The listing builds one solid part. Answer for the finished solid, in the listing's coordinates (mm). Face numbers are marked on the shaded views. A direction names the side the tool comes from. Coordinates: 2 decimals unless noted, no trailing zeros. Loops run counter-clockwise (first coordinate to the right, second up) from the corner with the lowest first, then second, coordinate; pieces in that order, holes last. Notation, with made-up numbers: (86, 74.5) - (136, 74.5) arc R18 cw to (136, 88.5) - close; hole circle Ø4 at (63.5, -26). An arc over 180 degrees is marked (long way). Write each question's results on one line, items separated by ' | '. Start each with the question number.
(1) Find section C-C on x = 7. Determine the outline of the cut face in (y, z), then the cut area to 3 significant figures.
(2) Find section A-A on y = 0. Determine the outline of the cut face in (x, z), then the cut area to 3 significant figures.
(3) Given pin 1 Ø12 at (x, y) = (-7, 30) entering from -Z; pin 2 Ø6 at (x, y) = (0, 35.5) entering from +Z; pin 3 Ø7 at (x, y) = (-17, 27.5) entering from +Z; pin 4 Ø3.5 at (x, y) = (-17, -27.5) entering from +Z, each flat-ended and moving along its own axis, determine where each tip first touches the part or whether it passes through.
(4) Consider line 1 (X direction, y = -27.5, z = 1.45); line 2 (Y direction, x = -27, z = -3.5); line 3 (Z direction, x = -29, y = -26.5). Determine where each line is inside the solid, lowest interval first. Write a range as from..to.
(5) Find section D-D on y = -17.75. Determine the outline of the cut face in (x, z), then the cut area to 3 significant figures.
(6) For the marked faces 1, 2 and 3, determine the directions among +Z, -Z, +X, -X, +Y, -Y from which every point of the face is accessible in a straight line to the end or side of a thin tool.
(7) Find section B-B on x = -17. Determine the outline of the cut face in (y, z).
(8) Determine the mould class of the marked faces 4, 5 and 6 for opening direction Y: released by +Y, released by -Y, zero draft, split by the parting line, or undercut.
from build123d import *

# Parameters (mm, degrees)
SKETCH_1_W                     = 80
SKETCH_1_H                     = 80
SKETCH_1_R                     = 25
EXTRUDE_1_DEPTH                = 6
SKETCH_11_W                    = 10
SKETCH_11_H                    = 10
EXTRUDE_3_DEPTH                = 10
HOLE_WIZARD_M4_1_D             = 4.5
HOLE_WIZARD_M4_1_CSINK_D       = 8.96
HOLE_WIZARD_M4_1_CSINK_ANGLE   = 90
HOLE_WIZARD_M4_2_D             = 3.3
HOLE_WIZARD_M4_2_DEPTH         = 68
MIRROR_2_COPY_1_SKETCH_W       = 10
MIRROR_2_COPY_1_SKETCH_H       = 10
MIRROR_2_COPY_1_DEPTH          = 10
MIRROR_2_COPY_2_D              = 3.3
MIRROR_2_COPY_2_DEPTH          = 68
HOLE_WIZARD_M4_1_2_D           = 4.5
HOLE_WIZARD_M4_1_2_CSINK_D     = 9.4
HOLE_WIZARD_M4_1_2_CSINK_ANGLE = 90
CHAMFER_1_SIZE                 = 1


with BuildPart() as part:
    # 스케치1 → 보스-돌출1 (new body)
    with BuildSketch(Plane.XY):
        Rectangle(SKETCH_1_W, SKETCH_1_H)
        Circle(SKETCH_1_R, mode=Mode.SUBTRACT)
    extrude(amount=EXTRUDE_1_DEPTH)

    # 스케치11 → 보스-돌출3 (add)
    with BuildSketch(Plane(origin=(0, 0, 0), x_dir=(-1, 0, 0), z_dir=(0, 0, -1))):
        with Locations((29, 29)):
            Rectangle(SKETCH_11_W, SKETCH_11_H)
    extrude_3 = extrude(amount=EXTRUDE_3_DEPTH)

    # Hole Wizard M4 _ _ _ _ _ _ _1 (through all)
    with Locations(Plane(origin=(0, 0, 0), x_dir=(-1, 0, 0), z_dir=(0, 0, -1))):
        with Locations((0, -35.5), (30.743901834, -17.75), (30.743901834, 17.75), (0, 35.5), (-30.743901834, 17.75), (-30.743901834, -17.75)):
            CounterSinkHole(HOLE_WIZARD_M4_1_D / 2, HOLE_WIZARD_M4_1_CSINK_D / 2, counter_sink_angle=HOLE_WIZARD_M4_1_CSINK_ANGLE)

    # M4 나사 구멍2
    with Locations(Plane(origin=(0, 34, 0), x_dir=(1, 0, 0), z_dir=(0, 1, 0))):
        with Locations((-29, 5)):
            hole_wizard_m4_2 = Hole(HOLE_WIZARD_M4_2_D / 2, depth=HOLE_WIZARD_M4_2_DEPTH)

    # 대칭 복사1: 보스-돌출3, M4 나사 구멍2 across plane
    add(extrude_3.mirror(Plane(origin=(0, 0, 0), x_dir=(0, 0, 1), z_dir=(1, 0, 0))))
    add(hole_wizard_m4_2.mirror(Plane(origin=(0, 0, 0), x_dir=(0, 0, 1), z_dir=(1, 0, 0))), mode=Mode.SUBTRACT)

    # 대칭 복사2: 보스-돌출3, M4 나사 구멍2 across plane
    add(extrude_3.mirror(Plane.ZX))
    add(hole_wizard_m4_2.mirror(Plane.ZX), mode=Mode.SUBTRACT)

    # 대칭 복사2 copy 1 sketch → 대칭 복사2 copy 1 (add)
    with BuildSketch(Plane(origin=(0, 0, 0), x_dir=(1, 0, 0), z_dir=(0, 0, -1))):
        with Locations((29, 29)):
            Rectangle(MIRROR_2_COPY_1_SKETCH_W, MIRROR_2_COPY_1_SKETCH_H)
    extrude(amount=MIRROR_2_COPY_1_DEPTH)

    # 대칭 복사2 copy 2
    with Locations(Plane(origin=(0, -34, 0), x_dir=(-1, 0, 0), z_dir=(0, -1, 0))):
        with Locations((-29, 5)):
            Hole(MIRROR_2_COPY_2_D / 2, depth=MIRROR_2_COPY_2_DEPTH)

    # Hole Wizard M4 _ _ _ _1 2 (through all)
    with Locations(Plane.XY.offset(6)):
        with Locations((17, 27.5), (17, -27.5), (-17, 27.5), (-17, -27.5)):
            CounterSinkHole(HOLE_WIZARD_M4_1_2_D / 2, HOLE_WIZARD_M4_1_2_CSINK_D / 2, counter_sink_angle=HOLE_WIZARD_M4_1_2_CSINK_ANGLE)

    # 모따기1
    chamfer_1_edges = [part.edges().sort_by_distance(p)[0] for p in [
        (-34, -34, -5),
        (-34, 34, -5),
        (34, 34, -5),
        (34, -34, -5),
    ]]
    chamfer(chamfer_1_edges, length=CHAMFER_1_SIZE)


solid = part.part
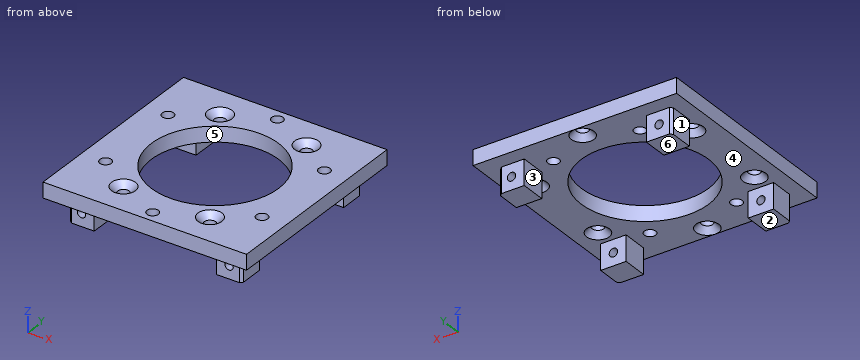
Values:
1) outline: (-40, 0) - (-24, 0) - (-24, 6) - (-40, 6) - close; (24, 0) - (40, 0) - (40, 6) - (24, 6) - close | area: 192 mm²
2) outline: (-40, 0) - (-25, 0) - (-25, 6) - (-40, 6) - close; (25, 0) - (40, 0) - (40, 6) - (25, 6) - close | area: 180 mm²
3) pin 1: stops at z = 0 | pin 2: stops at z = 6 | pin 3: stops at z = 4.8 | pin 4: passes through
4) line 1: x = -40..-19.25, -14.75..14.75, 19.25..40 | line 2: y = -34..-24, 24..34 | line 3: z = -10..-6.65, -3.35..6
5) outline: (-40, 0) - (-35.22, 0) - (-32.99, 2.23) - (-32.99, 6) - (-40, 6) - close; (-28.49, 2.23) - (-26.26, 0) - (-17.61, 0) - (-17.61, 6) - (-28.49, 6) - close; (17.61, 0) - (26.26, 0) - (28.49, 2.23) - (28.49, 6) - (17.61, 6) - close; (32.99, 2.23) - (35.22, 0) - (40, 0) - (40, 6) - (32.99, 6) - close | area: 205 mm²
6) face 1: -Z, -X, +Y, -Y | face 2: -Z, +X, -X, +Y, -Y | face 3: -Z, +Y, -Y
7) outline: (-40, 0) - (-29.75, 0) - (-29.75, 3.55) - (-32.2, 6) - (-40, 6) - close; (-25.25, 0) - (-18.33, 0) - (-18.33, 6) - (-22.8, 6) - (-25.25, 3.55) - close; (18.33, 0) - (25.25, 0) - (25.25, 3.55) - (22.8, 6) - (18.33, 6) - close; (29.75, 0) - (40, 0) - (40, 6) - (32.2, 6) - (29.75, 3.55) - close
8) face 4: undercut | face 5: undercut | face 6: zero draft
